Job drawing, mm, ordinate dimensions from the low corner. One solid piece. A direction names the side the tool comes from. Coordinates: 2 decimals unless noted, no trailing zeros. Order: outer loops, then holes, each group sorted by start corner. A loop starts at its lowest first (then second) coordinate and runs counter-clockwise, first axis right, second up. Notation, with made-up numbers: M -17,86 L 33,86 A15 cw 33,103 Z; hole C 89,5.25 d6. An arc over 180 degrees is marked long. Write item = value, one per line. Start each with the question number.
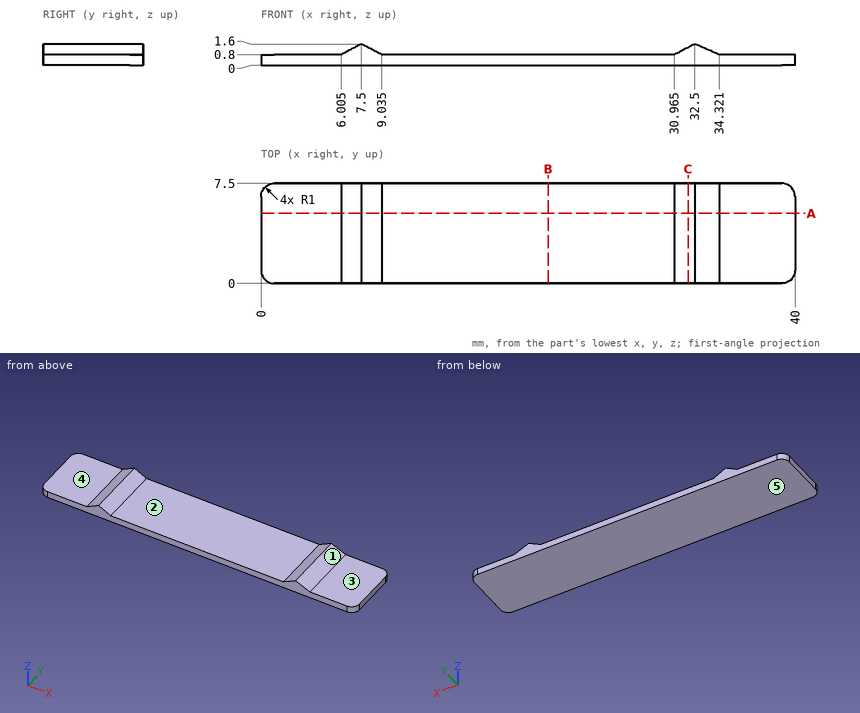
Item 1: Pull direction X, two halves, no side cores. Call the marked faces 1, 2 and 3: pulls with the +X half, pulls with the -X half, needs draft (parallel to the pull), parting line crosses it, or undercut.
Item 2: Flat gauge pin, fed straight in: pin 1 (4 mm diameter, centred on x = 20, y = 4, fed in from +Z). Where does the tip first touch, or does it go through?
Item 3: Cut at B-B, the plane x = 21.5. Write the cut outline in (y, z).
Item 4: 3-axis set-ups, long thin cutter, end or side, ignore diameter. For the marked faces 4 and 5: which of +Z, -Z, +X, -X, +Y, -Y reach the whole face in a straight line?
Item 5: Cut at A-A, the plane y = 5.25. Write the cut outline in (x, z) (1 decimal).
Item 6: Cut at C-C, the plane x = 32. Write the cut outline in (y, z).
Item 7: Wall check: line 1 along X through (y, z) = (5.25, 1.1) (1 decimal); line 2 along X through (y, z) = (7.25, 1.35) (1 decimal); line 3 along Z through (x, y) = (19, 7.25). Give the ranges that are in metal, low to high. Write a range as [from, to].
Filled sheet:
q1.face_1 = pulls with the +X half
q1.face_2 = undercut
q1.face_3 = needs draft
q2.pin_1 = 0.8
q3.outline = M 0,0 L 7.5,0 L 7.5,0.8 L 0,0.8 Z
q4.face_4 = +Z, -X, +Y, -Y
q4.face_5 = -Z, +X, -X, +Y, -Y
q5.outline = M 0,0 L 40,0 L 40,0.8 L 34.3,0.8 L 32.5,1.6 L 31,0.8 L 9,0.8 L 7.5,1.6 L 6,0.8 L 0,0.8 Z
q6.outline = M 0,0 L 7.5,0 L 7.5,1.34 L 0,1.34 Z
q7.line_1 = [6.6, 8.5], [31.5, 33.6]
q7.line_2 = [7, 8], [32, 33.1]
q7.line_3 = [0, 0.8]
